CAD build for the part. Positions are in the model's coordinates, mm. Round coordinates to 2 decimals unless told otherwise and drop trailing zeros. Order: outer loops, then holes, each group sorted by start corner. A loop starts at its lowest first (then second) coordinate and runs counter-clockwise, first axis right, second up. Notation, with made-up numbers: (-26.75, 62.5) - (27.25, 62.5) arc R20 cw to (27.25, 85.5) - close; hole circle Ø4 at (34, 86.5). An arc over 180 degrees is marked (long way). Use one line per item in the form item = value. Start each with the question number.
from build123d import *

# Parameters (mm, degrees)
SKETCH_1_W          = 34
SKETCH_1_H          = 11
EXTRUDE_1_DEPTH     = 1.6
SKETCH_2_R          = 1.4
CUT_EXTRUDE_2_DEPTH = 6.6
SKETCH_4_R          = 0.25
CUT_EXTRUDE_3_DEPTH = 10


with BuildPart() as part:
    # 草图1 → 拉伸1 (new body)
    with BuildSketch(Plane(origin=(0, 0, 0), x_dir=(1, 0, 0), z_dir=(0, 1, 0))):
        Rectangle(SKETCH_1_W, SKETCH_1_H)
    extrude(amount=EXTRUDE_1_DEPTH)

    # 草图2 → 切除-拉伸2 (cut)
    with BuildSketch(Plane(origin=(0, 0, 0), x_dir=(1, 0, 0), z_dir=(0, 1, 0))):
        with Locations(Location((-11, 0, 0), (0, 0, 270))):
            Circle(SKETCH_2_R)
        with Locations(Location((13.5, -2.7, 0), (0, 0, 270))):
            Circle(SKETCH_2_R)
    extrude(amount=CUT_EXTRUDE_2_DEPTH, mode=Mode.SUBTRACT)

    # 草图3 → 旋转1 (revolve)
    with BuildSketch(Plane.XY.offset(2.5)):
        with BuildLine():
            Line((0, 1.6), (-3, 1.6))
            Line((-3, 1.6), (-3, 2.060607986))
            ThreePointArc((-3, 2.060607986), (-1.482423007, 1.944785244), (0, 1.6))
        make_face()
    revolve(axis=Axis((-3, 10.072937712, 2.5), (0, -1, 0)))

    # 草图4 → 切除-拉伸3 (cut)
    with BuildSketch(Plane(origin=(0, 1.6, 0), x_dir=(-1, 0, 0), z_dir=(0, 1, 0))):
        with Locations(Location((3.2, -1.5, 0), (0, 0, 90))):
            Circle(SKETCH_4_R)
        with Locations(Location((0.66, -1.5, 0), (0, 0, 90))):
            Circle(SKETCH_4_R)
        with Locations(Location((-1.88, -1.5, 0), (0, 0, 90))):
            Circle(SKETCH_4_R)
        with Locations(Location((-4.42, -1.5, 0), (0, 0, 90))):
            Circle(SKETCH_4_R)
    extrude(amount=-CUT_EXTRUDE_3_DEPTH, mode=Mode.SUBTRACT)


solid = part.part
(1) Mould opens along X. For faces 1 (the cylindrical face through (-9.82, 0.79, 0.75)), 2 (the flat face through (0, 1.6, 0)), 3 (the flat face through (17, 1, 0)) say: pulls with the +X half, pulls with the -X half, needs draft (parallel to the pull), parting line crosses it, or undercut.
(2) Slice it at B-B (x = -11). Give the cut face in (y, z), and give its area (3 significant figures).
(3) Slice it at A-A (y = 0.3). Give the cut face in (x, z), and give its area (3 significant figures).
(4) Slice it at D-D (x = -4.5). Give the cut face in (y, z).
(5) Flat gauge pins, fed straight in: P1, Ø2, axis at x = -3, z = -2, coming from the +Y side; P2, Ø4.5, axis at x = 13.5, z = 2.7, coming from the -Y side. Where does each tip first touch, or does it go through?
(6) Slice it at C-C (z = 0). Give the cut face in (x, y), and give its area (3 significant figures).
(7) Wall check: line 1 (X direction, y = 0.55, z = -1.5); line 2 (X direction, y = 1.4, z = 2.75); line 3 (X direction, y = 0.5, z = 0). Give the ranges that are in metal, low to high. Write a range as [from, to].
Results list:
q1.face_1 = undercut
q1.face_2 = needs draft
q1.face_3 = pulls with the +X half
q2.outline = (0, -5.5) - (1.6, -5.5) - (1.6, -1.4) - (0, -1.4) - close; (0, 1.4) - (1.6, 1.4) - (1.6, 5.5) - (0, 5.5) - close
q2.area = 13.1 mm²
q3.outline = (-17, -5.5) - (17, -5.5) - (17, 5.5) - (-17, 5.5) - close; hole circle Ø2.8 at (-11, 0); hole circle Ø0.5 at (-3.2, -1.5); hole circle Ø0.5 at (-0.66, -1.5); hole circle Ø0.5 at (1.88, -1.5); hole circle Ø0.5 at (4.42, -1.5); hole circle Ø2.8 at (13.5, 2.7)
q3.area = 361 mm²
q4.outline = (0, -5.5) - (1.6, -5.5) - (1.6, -0.1) arc R9.89 ccw to (1.6, 5.1) - (1.6, 5.5) - (0, 5.5) - close
q5.P1 = 1.6
q5.P2 = 0
q6.outline = (-17, 0) - (-12.4, 0) - (-12.4, 1.6) - (-17, 1.6) - close; (-9.6, 0) - (17, 0) - (17, 1.6) - (-1.34, 1.6) arc R9.68 ccw to (-4.66, 1.6) - (-9.6, 1.6) - close
q6.area = 50.2 mm²
q7.line_1 = [-17, -3.45], [-2.95, -0.91], [-0.41, 1.63], [2.13, 4.17], [4.67, 17]
q7.line_2 = [-17, 12.1], [14.9, 17]
q7.line_3 = [-17, -12.4], [-9.6, 17]
